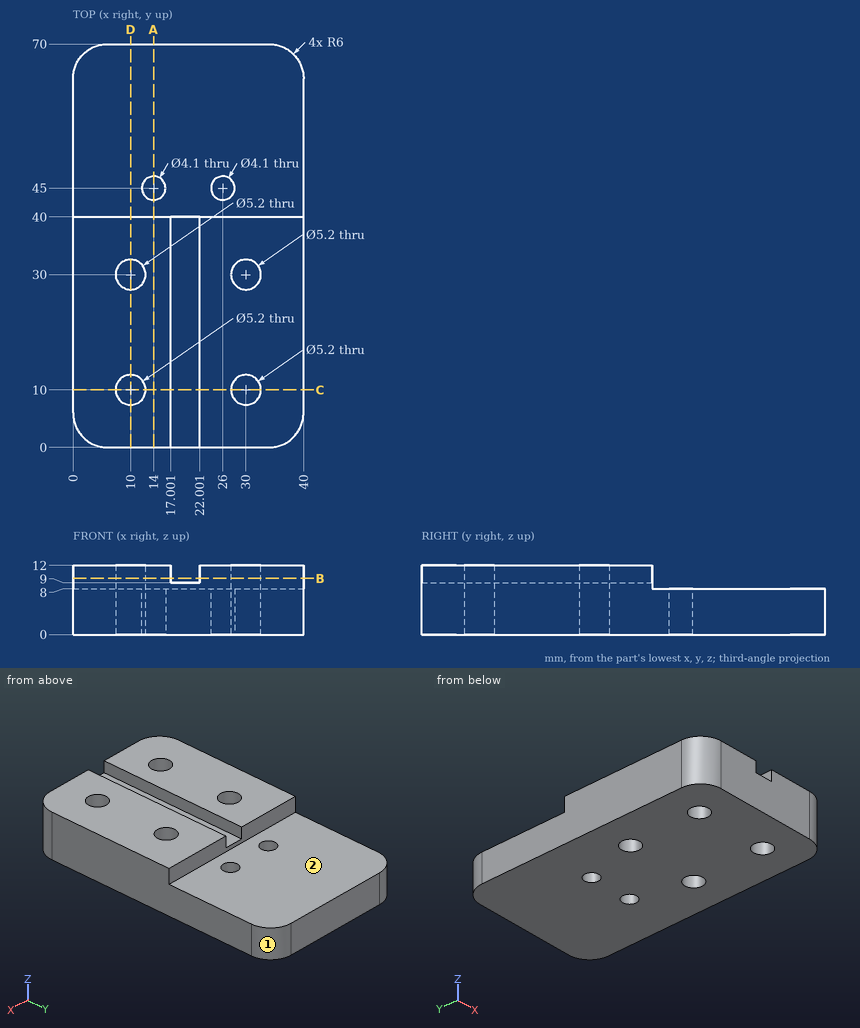
The figure shows three views and two pictorial views of one solid part (mm, origin at its lowest corner). Answer the questions. A direction names the side the tool comes from. Coordinates: 2 decimals unless noted, no trailing zeros. Loops run counter-clockwise (first coordinate to the right, second up) from the corner with the lowest first, then second, coordinate; pieces in that order, holes last. Notation, with made-up numbers: M 2,65.25 L 41,65.25 A30 ccw 41,94.25 Z; hole C 71,38.25 d2. An arc over 180 degrees is marked long. Use CSV: the item, a comma, the result in double quotes. Start each with the question number.
(1) Find section D-D, the plane x = 10. Give the vertices of the cut face in (y, z).
(2) Find section A-A, the plane x = 14. Give the vertices of the cut face in (y, z), then the cut area to 3 significant figures.
(3) Consider line 1 (Y direction, x = 30, z = 6.5); line 2 (Y direction, x = 31, z = 1.25); line 3 (Y direction, x = 26, z = 2). Determine where each line is inside the solid, lowest interval first.
(4) Find section B-B, the plane z = 9.75. Give the vertices of the cut face in (x, y), then the cut area to 3 significant figures.
(5) Find section C-C, the plane y = 10. Give the vertices of the cut face in (x, z), then the cut area to 3 significant figures.
(6) For the marked faces 1 and 2, determine the directions among +Z, -Z, +X, -X, +Y, -Y from which every point of the face is accessible in a straight line to the end or side of a thin tool.
(7) Given pin 1 Ø1.5 at (x, y) = (20.5, 22.5) entering from +Z; pin 2 Ø5.5 at (x, y) = (14, 45) entering from +Z; pin 3 Ø3 at (x, z) = (22, 10.5) entering from +Y, each flat-ended and moving along its own axis, determine where each tip first touches the part or whether it passes through.
Recorded:
1,outline,"M 0,0 L 7.4,0 L 7.4,12 L 0,12 Z; M 12.6,0 L 27.4,0 L 27.4,12 L 12.6,12 Z; M 32.6,0 L 70,0 L 70,8 L 40,8 L 40,12 L 32.6,12 Z"
2,outline,"M 0,0 L 42.95,0 L 42.95,8 L 40,8 L 40,12 L 0,12 Z; M 47.05,0 L 70,0 L 70,8 L 47.05,8 Z"
2,area,"687 mm^2"
3,line 1,"y = 0 to 7.4, 12.6 to 27.4, 32.6 to 70"
3,line 2,"y = 0 to 7.6, 12.4 to 27.6, 32.4 to 70"
3,line 3,"y = 0 to 42.95, 47.05 to 70"
4,outline,"M 0,6 A6 ccw 6,0 L 17,0 L 17,40 L 0,40 Z; M 22,0 L 34,0 A6 ccw 40,6 L 40,40 L 22,40 Z; hole C 10,10 d5.2; hole C 10,30 d5.2; hole C 30,10 d5.2; hole C 30,30 d5.2"
4,area,"1,300 mm^2"
5,outline,"M 0,0 L 7.4,0 L 7.4,12 L 0,12 Z; M 12.6,0 L 27.4,0 L 27.4,12 L 22,12 L 22,9 L 17,9 L 17,12 L 12.6,12 Z; M 32.6,0 L 40,0 L 40,12 L 32.6,12 Z"
5,area,"340 mm^2"
6,face 1,"+Z, -Z, +X, +Y"
6,face 2,"+Z, +X, -X, +Y"
7,pin 1,"stops at z = 9"
7,pin 2,"stops at z = 8"
7,pin 3,"stops at y = 40"
